Geometry check sheet. Reference: the model listing, model coordinates, mm. Face numbers are marked on the shaded views. A direction names the side the tool comes from. Coordinates: 2 decimals unless noted, no trailing zeros. Write each loop counter-clockwise with the first axis right and the second up, starting at its lowest first coordinate (ties: lowest second). Pieces come first, ordered by that corner, then holes. Notation, with made-up numbers: M 83,50 L 113,50 A21 cw 113,75 Z; hole C 83.25,6.5 d6. An arc over 180 degrees is marked long. Put each result on its own line as item: value. Start each with the question number.
1) Cross-section at A-A on z = 13.75. Count the separate pieces of the cut face and the enclosed holes in it, plus the area to 3 significant figures.
2) Cross-section at C-C on x = -1. Record the cut outline in (y, z) (3 decimals), plus the area to 3 significant figures.
3) Gauge pin test, flat ends, axial feed: pin 1 (5.5 mm diameter, centred on y = -2.5, z = 8, fed in from +X); pin 2 (2 mm diameter, centred on x = 3, y = 1, fed in from +Z) (3 decimals). Record the tip position at first contact, or that the pin passes through.
4) Scan line: line 1 along Z through (x, y) = (-5.5, 8) (3 decimals). Record every from-to range of solid material in increasing order.
5) Set-up check for the marked faces 1 and 2: record each of +Z, -Z, +X, -X, +Y, -Y from which the full face is reachable in a straight line by a thin tool's end or side.
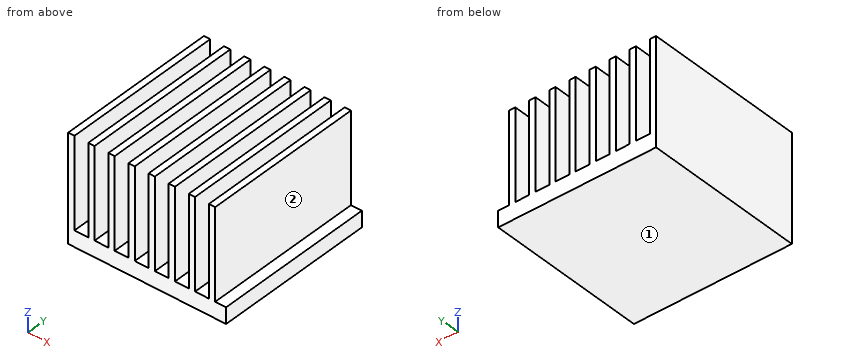
from build123d import *

# Parameters (mm, degrees)
SKETCH1_W           = 31.42
SKETCH1_H           = 32
BOSS_EXTRUDE1_DEPTH = 3.175
SKETCH2_W           = 1.25
SKETCH2_H           = 32
BOSS_EXTRUDE2_DEPTH = 18
LPATTERN1_COUNT     = 8
LPATTERN1_PITCH     = 4


with BuildPart() as part:
    # Sketch1 → Boss-Extrude1 (new body)
    with BuildSketch(Plane.XY):
        Rectangle(SKETCH1_W, SKETCH1_H)
    extrude(amount=BOSS_EXTRUDE1_DEPTH)

    # Sketch2 → Boss-Extrude2 (add)
    with BuildSketch(Plane.XY.offset(3.175)):
        with Locations((-15.085, 0)):
            Rectangle(SKETCH2_W, SKETCH2_H)
    boss_extrude2 = extrude(amount=BOSS_EXTRUDE2_DEPTH)

    # LPattern1: Boss-Extrude2 ×8
    with Locations(*[(i * LPATTERN1_PITCH, 0, 0) for i in range(1, LPATTERN1_COUNT)]):
        add(boss_extrude2)


solid = part.part
Answer key:
1. separate pieces: 8
1. enclosed holes: 0
1. area: 320 mm²
2. outline: M -16,0 L 16,0 L 16,3.175 L -16,3.175 Z
2. area: 102 mm²
3. pin 1: stops at x = 13.54
3. pin 2: stops at z = 3.175
4. line 1: z = 0 to 3.175
5. face 1: -Z, +X, -X, +Y, -Y
5. face 2: +Z, +X, +Y, -Y
